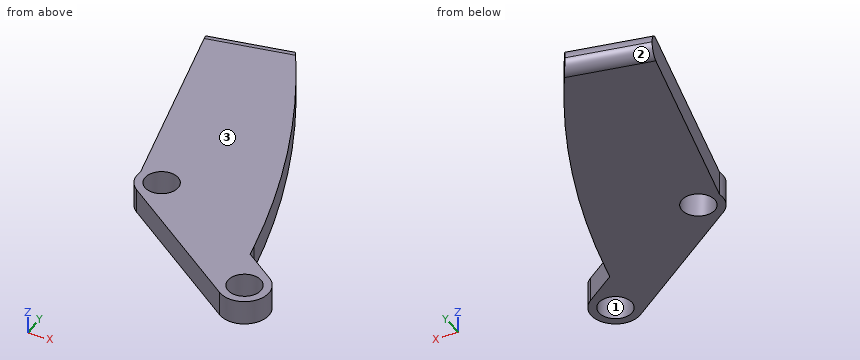
```python
from build123d import *

# Parameters (mm, degrees)
SKETCH1_R           = 2.7
BOSS_EXTRUDE1_DEPTH = 4
BOSS_EXTRUDE2_DEPTH = 4
FILLET4_R           = 150
FILLET5_R           = 2


# Some blends are built 0.0001 mm under size
with BuildPart() as part:
    # Sketch1 → Boss-Extrude1 (new body)
    with BuildSketch(Plane.XY):
        with BuildLine():
            Line((-24.747899147, 13.14945447), (-2.361821958, -3.228280818))
            ThreePointArc((-2.361821958, -3.228280818), (3.228280818, -2.361821958), (2.361821958, 3.228280818))
            Line((2.361821958, 3.228280818), (-20.024255231, 19.606016105))
            ThreePointArc((-20.024255231, 19.606016105), (-25.614358007, 18.739557246), (-24.747899147, 13.14945447))
        make_face()
        Circle(SKETCH1_R, mode=Mode.SUBTRACT)
        with Locations((-22.386077189, 16.377735287)):
            Circle(SKETCH1_R, mode=Mode.SUBTRACT)
    extrude(amount=BOSS_EXTRUDE1_DEPTH)

    # Sketch2 → Boss-Extrude2 (add, through all)
    with BuildSketch(Plane.XY.offset(4)):
        with BuildLine():
            Line((-26.299706155, 17.204480908), (-34.069064165, 52.206086792))
            Line((-34.069064165, 52.206086792), (-21.14349971, 54.723244673))
            Line((-21.14349971, 54.723244673), (-13.231740333, 56.386597335))
            Line((-13.231740333, 56.386597335), (-2.8588348, 7.047732243))
            Line((-2.8588348, 7.047732243), (-13.354395565, 14.726322576))
            Line((-13.354395565, 14.726322576), (-20.024255231, 19.606016105))
            ThreePointArc((-20.024255231, 19.606016105), (-23.81571668, 20.113525823), (-26.299706155, 17.204480908))
        make_face()
    extrude(amount=-BOSS_EXTRUDE2_DEPTH)

    # Fillet4
    # the kernel refuses this fillet: 150 mm, written as the material it takes off along each edge
    with BuildSketch(Plane(origin=(-13.231740333, 56.386597335, 125.450940965), x_dir=(0.20574032293470337, -0.9786066214361745, 0), z_dir=(0, 0, -1))) as fillet4_piece_1:
        with BuildLine():
            CenterArc((48.580376386, 150), FILLET4_R, 251.102921571, 18.897078429)
            Line((0, 8.084718828), (0, 0))
            Line((0, 0), (48.580376386, 0))
        make_face()
    extrude(amount=246.90188193, mode=Mode.SUBTRACT)

    # Fillet5
    fillet5_edges = [part.edges().sort_by_distance(p)[0] for p in [
        (-27.606281937, 53.464665733, 4),
        (-27.606281937, 53.464665733, 0),
    ]]
    fillet(fillet5_edges, radius=FILLET5_R - 0.0001)  # a hair under: the kernel refuses the full size


solid = part.part
```
Input: part model. Units: mm. Frame: model coordinates. Face numbers are marked on the shaded views. Coordinates: 2 decimals unless noted, no trailing zeros. Loops run counter-clockwise (first coordinate to the right, second up) from the corner with the lowest first, then second, coordinate; pieces in that order, holes last. Notation, with made-up numbers: (68, 52) -> (119, 52) arc R29 ccw to (119, 75) -> close; hole circle Ø2 at (54, 38.25). An arc over 180 degrees is marked (long way). Use a Markdown table: item, result.
1) Cut plane D-D (y = 30.5). Return the cut outline in (x, z), then the cut area to 3 significant figures.
Results found:
| item | result |
|---|---|
| outline | (-29.25, 0) -> (-9.52, 0) -> (-9.52, 4) -> (-29.25, 4) -> close |
| area | 78.9 mm2 |
2) Cut plane B-B (y = 0). Return the cut outline in (x, z), then the cut area to 3 significant figures.
Results found:
| item | result |
|---|---|
| outline | (-6.77, 0) -> (-2.7, 0) -> (-2.7, 4) -> (-6.77, 4) -> close; (2.7, 0) -> (4, 0) -> (4, 4) -> (2.7, 4) -> close |
| area | 21.5 mm2 |
3) Cut plane A-A (x = 0). Return the cut outline in (y, z).
Results found:
| item | result |
|---|---|
| outline | (-4, 0) -> (-2.7, 0) -> (-2.7, 4) -> (-4, 4) -> close; (2.7, 0) -> (4.96, 0) -> (4.96, 4) -> (2.7, 4) -> close |
4) Material intervals for line 1 along Y through (x, z) = (0, 1.15); line 2 along Y through (x, z) = (-24, 2.25); line 3 along X through (y, z) = (42.5, 2.2), sorted ascending. Write a range as from..to.
Results found:
| item | result |
|---|---|
| line 1 | y = -4..-2.7, 2.7..4.96 |
| line 2 | y = 12.6..14.21, 18.54..54.15 |
| line 3 | x = -31.91..-14.61 |
5) Contact query for flat-ended pins moving along their axis: pin 1 (2 mm diameter, centred on x = -22.5, z = 1.5, fed in from -Y); pin 2 (2 mm diameter, centred on y = 22, z = 3.5, fed in from +X). Output: stop coordinate, or through.
Results found:
| item | result |
|---|---|
| pin 1 | stops at y = 10.77 |
| pin 2 | stops at x = -6.33 |
6) Cut plane C-C (z = 0.6). Return the cut outline in (x, y), then the cut area to 3 significant figures.
Results found:
| item | result |
|---|---|
| outline | (-33.95, 51.65) -> (-26.3, 17.2) arc R4 ccw to (-24.75, 13.15) -> (-2.36, -3.23) arc R4 ccw to (2.36, 3.23) -> (-2.86, 7.05) -> (-3.24, 8.85) arc R150 ccw to (-20.83, 54.2) -> close; hole circle Ø5.4 at (-22.39, 16.38); hole circle Ø5.4 at (0, 0) |
| area | 926 mm2 |
7) Pull-direction query (X, two-part tool) for the marked faces 1, 2 and 3; classes: released by +X, released by -X, zero draft, split by the parting line, or undercut.
Results found:
| item | result |
|---|---|
| face 1 | undercut |
| face 2 | released by -X |
| face 3 | zero draft |
